Study the drawing (mm; zero at the part's minimum x, y, z) and answer. A direction names the side the tool comes from. Coordinates: 2 decimals unless noted, no trailing zeros. One line per item, written item: value.
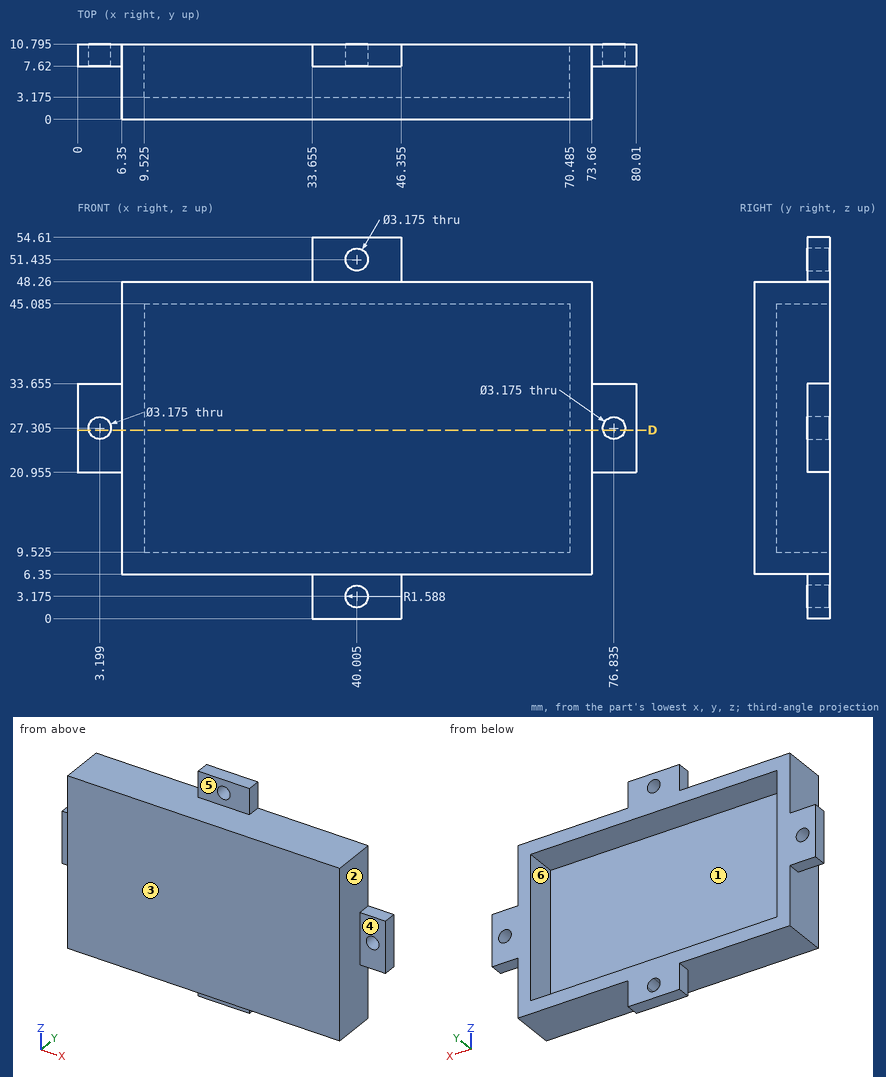
Item 1: Given pin 1 (3.5 mm diameter, centred on y = 9, z = 50.5, fed in from +X) (1 decimal); pin 2 (5 mm diameter, centred on x = 40.005, z = 51.435, fed in from -Y); pin 3 (2.5 mm diameter, centred on x = 47.5, y = 7, fed in from -Z); pin 4 (7 mm diameter, centred on x = 41.5, z = 50, fed in from -Y), each flat-ended and moving along its own axis, determine where each tip first touches the part or whether it passes through.
Evaluation:
pin 1: stops at x = 46.4
pin 2: stops at y = 7.62
pin 3: stops at z = 6.35
pin 4: stops at y = 0
Item 2: Section D-D, the plane z = 27 is taken. Give the number of separate pieces and of enclosed holes in the cut face.
Evaluation:
separate pieces: 3
enclosed holes: 0
Item 3: Which of the six approach directions +Z, -Z, +X, -X, +Y, -Y give full straight-line access (tool end or side, diameter ignored) to the marked faces 3, 4, 5 and 6?
Evaluation:
face 3: +Z, -Z, +X, -X, -Y
face 4: +Z, -Z, +X, -Y
face 5: +Z, +X, -X, -Y
face 6: +Y
Item 4: Consider probe 1 along Z at (x, y) = (38, 9.5) (1 decimal); probe 2 along X at (y, z) = (9.5, 32.5) (1 decimal); probe 3 along Y at (x, z) = (31, 11.5) (1 decimal). Determine where each line is inside the solid, lowest interval first.
Evaluation:
probe 1: z = 0 to 9.5, 45.1 to 54.6
probe 2: x = 0 to 9.5, 70.5 to 80
probe 3: y = 0 to 3.2
Item 5: Determine the mould class of the marked faces 1 and 2 for opening direction Z: +Z half, -Z half, draft (parallel to the pull), parting line (faces both ways), or undercut.
Evaluation:
face 1: undercut
face 2: draft
